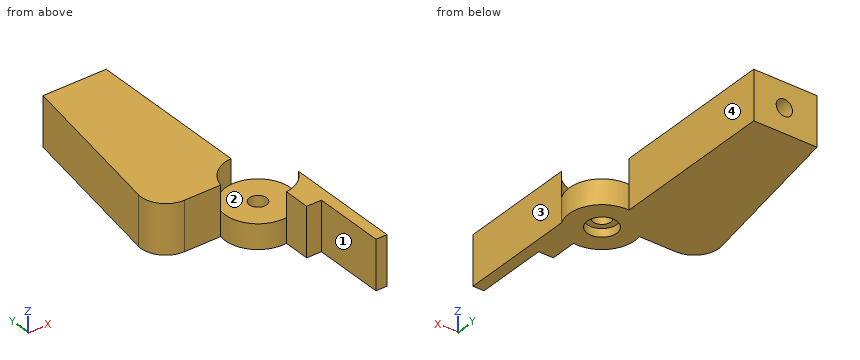
Autodesk Inventor part; units mm, degrees
ref_plane "YZ Plane" through (0, 0, 0) normal (1, 0, 0) x (0, 1, 0)
ref_plane "XZ Plane" through (0, 0, 0) normal (0, 1, 0) x (-1, 0, 0)
ref_plane "XY Plane" through (0, 0, 0) normal (0, 0, 1) x (1, 0, 0)
sketch "Sketch1" plane through (0, 0, 0) normal (0, 0, 1) x (1, 0, 0)
  circle A0 centre (0, 0) radius 4
  line L0 (0, 24) -> (-8, 24)
  line L1 (0, 24) -> (0, 4)
  line L2 (-11.9043, 0.8695) -> (-3.9043, 0.8695)
  line L3 (-11.9043, 0.8695) -> (-8, 24)
  dimension "d9" = 6
  dimension "d0" = 8
  dimension "d6" = 8
  dimension "d94" = 20
  dimension "d95" = 8
extrude "Extrusion1" add sketch "Sketch1" along normal mid plane 6
sketch "Sketch2" plane through (0, 0, 3) normal (0, 0, 1) x (1, 0, 0)
  circle A0 centre (0, 0) radius 4
extrude "Extrusion2" cut sketch "Sketch2" against normal blind 3
sketch "Sketch4" plane through (-8, 24, 3) normal (0, 1, 0) x (1, 0, 0)
  line L0 (8, 6) -> (8, 0)
  line L1 (0, 0) -> (8, 6)
  line L2 (8, 0) -> (0, 0)
  line L3 (0, 6) -> (0, 0)
  line L4 (8, 0) -> (0, 6)
  circle A0 centre (4, 3) radius 1
  point P0 (8, 3)
  point P1 (3.2, 2.4)
  point P2 (3.2, 3.6)
  dimension "d9" = 6
  dimension "d17" = 2
  dimension "d93" = 1.2
extrude "Extrusion4" cut sketch "Sketch4" against normal blind 5 contours A0 L4 L1 | L1 L4 A0 | A0 L1 L4 | L1 A0 L4
sketch "Sketch8" plane through (0, 0, 0) normal (0, 0, 1) x (1, 0, 0)
  arc A0 (-3.9043, 0.8695) -> (0, 4) centre (0, 0) ccw
  dimension "d9" = 6
hole "Hole3" at (0, 0, 0) direction (0, 0, -1) diameter 2.1 end through all
sketch "Sketch9" plane through (0, 0, 0) normal (0, 0, 1) x (1, 0, 0)
  line L0 (0, 4) -> (0, 24) construction
  line L1 (0, 24) -> (-8, 24) construction
  line L2 (-3.2679, 22.7321) -> (-9.3121, 0.175) construction
  line L3 (-11.9043, 0.8695) -> (-3.9043, 0.8695) construction
  arc A0 (0, 4) -> (-3.9043, 0.8695) centre (0, 0) ccw construction
  arc A1 (-3.9043, 0.8695) -> (0, 4) centre (0, 0) ccw
  line L4 (0, 31.995) -> (0, -23.9701) construction
  arc A2 (-3.9043, 0.8695) -> (0, 4) centre (0, 0) ccw construction
  line L5 (0.446, -3.9751) -> (0.446, -10.9751)
  line L6 (3.846, -1.0991) -> (3.846, -15.9751)
  line L7 (0.446, -10.9751) -> (2.246, -10.9751)
  line L8 (2.246, -10.9751) -> (2.246, -15.9751)
  line L9 (2.246, -15.9751) -> (3.846, -15.9751)
  point P0 (0.446, -3.9751)
  dimension "d9" = 6
  dimension "d90" = 7
  dimension "d91" = 3.4
  dimension "d92" = 1.8
extrude "Extrusion5" add sketch "Sketch9" along normal mid plane 6
sketch "Sketch10" plane through (0, 0, -3) normal (0, 0, -1) x (-1, 0, 0)
  circle A0 centre (0, 0) radius 1.05
  circle A1 centre (0, 0) radius 1.8
  dimension "d9" = 6
  dimension "d62" = 3.6
extrude "Extrusion6" cut sketch "Sketch10" against normal blind 1
fillet "Fillet2" radius 3 1 edges at (-11.9043, 0.8695, 0)
move faces "Move1" translate (-0.25, 0, 0) faces at (3.846, -11.0164, 0)
move faces "Move2" translate (-0.25, 0, 0) faces at (0, 17.3333, 0)
move faces "Move3" translate (0, 3.75, 0) faces at (1.646, -10.9751, 1)
properties part number "pliers" material "ABS Plastic"
Source: CAD feature listing. Evaluate the final solid. Frame: model axes, mm. Face numbers are marked on the shaded views. A direction names the side the tool comes from. Coordinates: 2 decimals unless noted, no trailing zeros. Write each loop counter-clockwise with the first axis right and the second up, starting at its lowest first coordinate (ties: lowest second). Pieces come first, ordered by that corner, then holes. Notation, with made-up numbers: (-15.5, 71.5) -> (1.5, 71.5) arc R12 cw to (1.5, 76.5) -> close; hole circle Ø11 at (12.5, 56.25). An arc over 180 degrees is marked (long way). Return JSON: item names as keys, results as strings. Group by question number.
1) Section query D-D, the plane y = -4.5. Return loops of the section in (x, z), plus the area to 3 significant figures.
2) Section query B-B, the plane z = 0.5. Return loops of the section in (x, y), plus the area to 3 significant figures.
3) Section query C-C, the plane x = -5.5. Return loops of the section in (y, z).
4) Contact query for flat-ended pins moving along their axis: P1, Ø3.5, axis at y = -5, z = 0, coming from the -X side; P2, Ø3, axis at y = 18.5, z = 0.5, coming from the +X side; P3, Ø1.2, axis at x = -4, z = 0, coming from the -Y side; P4, Ø1.9, axis at x = 0, y = 0, coming from the -Z side. Output: stop coordinate, or through.
5) Section query A-A, the plane y = 0. Return loops of the section in (x, z), plus the area to 3 significant figures.
6) Ray query, line 1 along Y through (x, z) = (0, -0.6); line 2 along Z through (x, y) = (-4, 21.8); line 3 along Y through (x, z) = (0, -2.15). Return the intervals inside material, ascending.
7) Set-up query: the marked faces 1, 2, 3 and 4. Return all of +Z, -Z, +X, -X, +Y, -Y with unobstructed straight access to the full face (end or side cutting, diameter ignored); none if empty.
From the geometry:
{
 "1": {"outline": "(0.45, -3) -> (3.6, -3) -> (3.6, 3) -> (0.45, 3) -> close", "area": "18.9 mm²"},
 "2": {"outline": "(-11.31, 4.37) arc R3 ccw to (-8.36, 0.87) -> (-3.9, 0.87) arc R4 cw to (-0.25, 3.99) -> (-0.25, 24) -> (-3.13, 24) -> (-3.13, 19) -> (-4.87, 19) -> (-4.87, 24) -> (-8, 24) -> close; (0.45, -7.23) -> (2.25, -7.23) -> (2.25, -15.98) -> (3.6, -15.98) -> (3.6, -1.75) arc R4 cw to (0.45, -3.97) -> close", "area": "229 mm²"},
 "3": {"outline": "(0.87, -3) -> (24, -3) -> (24, 3) -> (0.87, 3) -> close"},
 "4": {"P1": "x = -2.33", "P2": "x = -0.25", "P3": "y = -2.11", "P4": "through"},
 "5": {"outline": "(-4, -3) -> (-1.8, -3) -> (-1.8, -2) -> (-1.05, -2) -> (-1.05, 0) -> (-4, 0) -> close; (1.05, -2) -> (1.8, -2) -> (1.8, -3) -> (4, -3) -> (4, 0) -> (1.05, 0) -> close", "area": "16.2 mm²"},
 "6": {"line 1": "-4 to -1.05, 1.05 to 4", "line 2": "-3 to -1, 1 to 3", "line 3": "-4 to -1.8, 1.8 to 4"},
 "7": {"face 1": "+Z, -Z, -X, -Y", "face 2": "+Z", "face 3": "+Z, -Z, +X, -Y", "face 4": "+Z, -Z, +X, +Y"}
}
